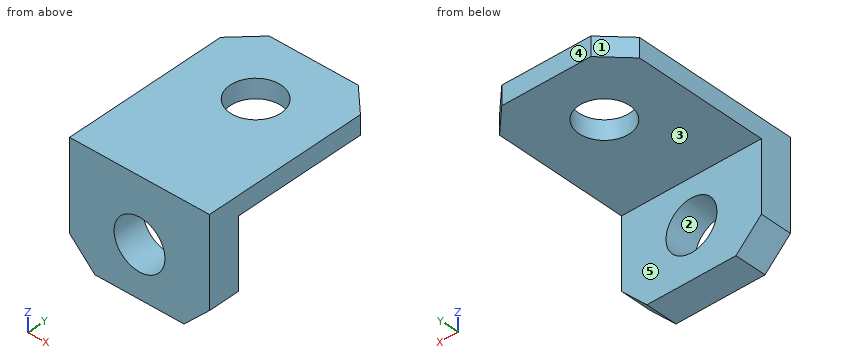
from build123d import *

# Parameters (mm, degrees)
SKETCH_1_W      = 22
SKETCH_1_H      = 18
SKETCH_1_R      = 4
EXTRUDE_1_DEPTH = 5
SKETCH_2_W      = 22
SKETCH_2_H      = 25
SKETCH_2_R      = 4
EXTRUDE_2_DEPTH = 3
CHAMFER_1_SIZE  = 4


with BuildPart() as part:
    # 草图1 → 凸台-拉伸1 (new body)
    with BuildSketch(Plane(origin=(0, 0, 0), x_dir=(1, 0, 0), z_dir=(0, 1, 0))):
        with Locations((-0.467181467, -2.976833977)):
            Rectangle(SKETCH_1_W, SKETCH_1_H)
        with Locations(Location((-0.467181467, -1.976833977, 0), (0, 0, 270))):
            Circle(SKETCH_1_R, mode=Mode.SUBTRACT)
    extrude(amount=EXTRUDE_1_DEPTH)

    # 草图2 → 凸台-拉伸2 (add)
    with BuildSketch(Plane.XY.offset(11.976833977)):
        with Locations((-0.467181467, 17.5)):
            Rectangle(SKETCH_2_W, SKETCH_2_H)
        with Locations((-0.467181467, 20)):
            Circle(SKETCH_2_R, mode=Mode.SUBTRACT)
    extrude(amount=-EXTRUDE_2_DEPTH)

    # 倒角1
    chamfer_1_edges = [part.edges().sort_by_distance(p)[0] for p in [
        (-11.467181467, 30, 10.476833977),
        (10.532818533, 30, 10.476833977),
        (-11.467181467, 2.5, -6.023166023),
        (10.532818533, 2.5, -6.023166023),
    ]]
    chamfer(chamfer_1_edges, length=CHAMFER_1_SIZE)


solid = part.part
Model file for the job. Use its own axes, mm. Face numbers are marked on the shaded views. A direction names the side the tool comes from. Give positions to 0.01 mm unless a question says otherwise; leave off trailing zeros. Write each loop counter-clockwise with the first axis right and the second up, starting at its lowest first coordinate (ties: lowest second). Pieces come first, ordered by that corner, then holes. Notation, with made-up numbers: (-11.5, -38.5) - (46.5, -38.5) arc R21 ccw to (46.5, -33.5) - close; hole circle Ø1 at (38.25, -4). An arc over 180 degrees is marked (long way). Answer as CSV lines item,"result".
1. Two-plate mould, pull along X, no slides. Class the marked faces 1, 2 and 3: +X half, -X half, draft (parallel to the pull), parting line (faces both ways), or undercut.
Responses:
face 1,"-X half"
face 2,"undercut"
face 3,"draft"
2. Band-saw the part on A-A (y = 20). Write the cut outline in (x, z).
Responses:
outline,"(-11.47, 8.98) - (-4.47, 8.98) - (-4.47, 11.98) - (-11.47, 11.98) - close; (3.53, 8.98) - (10.53, 8.98) - (10.53, 11.98) - (3.53, 11.98) - close"
3. Band-saw the part on D-D (z = 0). Write the cut outline in (x, y), and give its area (3 significant figures).
Responses:
outline,"(-11.47, 0) - (-3.94, 0) - (-3.94, 5) - (-11.47, 5) - close; (3.01, 0) - (10.53, 0) - (10.53, 5) - (3.01, 5) - close"
area,"75.2 mm2"
4. Band-saw the part on B-B (z = 10.25). Write the cut outline in (x, y), and give its area (3 significant figures).
Responses:
outline,"(-11.47, 0) - (10.53, 0) - (10.53, 26) - (6.53, 30) - (-7.47, 30) - (-11.47, 26) - close; hole circle Ø8 at (-0.47, 20)"
area,"594 mm2"
5. Pin check, flat tips, straight feed: pin 1 (1.5 mm diameter, centred on x = -6.5, y = 19, fed in from -Z); pin 2 (10 mm diameter, centred on y = 25, z = 2, fed in from -X); pin 3 (3 mm diameter, centred on x = -6.5, z = 8, fed in from +Y). Stop position of each tip, or through.
Responses:
pin 1,"stops at z = 8.98"
pin 2,"passes through"
pin 3,"stops at y = 30"
6. 3-axis set-ups, long thin cutter, end or side, ignore diameter. For the marked faces 4 and 5: which of +Z, -Z, +X, -X, +Y, -Y reach the whole face in a straight line?
Responses:
face 4,"+Z, -Z, +X, -X, +Y"
face 5,"-Z, +X, -X, +Y"
7. Band-saw the part on C-C (x = -9.25). Write the cut outline in (y, z).
Responses:
outline,"(0, -4.24) - (5, -4.24) - (5, 8.98) - (28.22, 8.98) - (28.22, 11.98) - (0, 11.98) - close"
8. Drill centre lines: L1, parallel to Z at x = 9.25, y = 9.5; L2, parallel to Y at x = 3.75, z = 5.25; L3, parallel to X at y = 23, z = 9.25. Where is each one in solid material? Low to high. Write a range as [from, to].
Responses:
L1,"z = [8.98, 11.98]"
L2,"y = [0, 5]"
L3,"x = [-11.47, -3.11], [2.18, 10.53]"
